Input: part model. Units: mm. Frame: model coordinates. Face numbers are marked on the shaded views. Give positions to 0.01 mm unless a question says otherwise; leave off trailing zeros. Write each loop counter-clockwise with the first axis right and the second up, starting at its lowest first coordinate (ties: lowest second). Pieces come first, ordered by that corner, then holes. Notation, with made-up numbers: (-37.75, -7.75) - (-11.75, -7.75) arc R15 cw to (-11.75, 15.25) - close; hole circle Ø4 at (-17, -19). An arc over 180 degrees is marked (long way). Use a Markdown table: item, result. Add a question column.
1. Section query A-A, the plane y = 0. Return loops of the section in (x, z), plus the area to 3 significant figures.
2. Pin query (flat end, axial travel): pin 1 (2 mm diameter, centred on x = -4.5, y = -12, fed in from -Z); pin 2 (1 mm diameter, centred on x = 3.5, z = -15, fed in from +Y); pin 3 (3 mm diameter, centred on x = 6.5, y = 30.5, fed in from -Z). Return the tip coordinate at first contact, or that it passes through.
3. Mould query, pull axis Y, two halves, no side actions, for the marked faces 1, 2 and 3. Classes: released by +Y, released by -Y, zero draft, split by the parting line, or undercut.
4. Section query C-C, the plane x = -4.5. Return loops of the section in (y, z), plus the area to 3 significant figures.
5. Material intervals for probe 1 along Y at (x, z) = (-1.5, 0); probe 2 along Y at (x, z) = (-6, -5); probe 3 along Z at (x, y) = (-6, -9.5), sorted ascending.
```python
from build123d import *

# Parameters (mm, degrees)
SKETCH1_R           = 39.5
SKETCH1_R_2         = 25
BOSS_EXTRUDE1_DEPTH = 8.75
FILLET1_R           = 3
CHAMFER1_SIZE       = 1.3


with BuildPart() as part:
    # Sketch1 → Boss-Extrude1 (new, symmetric)
    with BuildSketch(Plane(origin=(0, 0, 0), x_dir=(0, 0, -1), z_dir=(1, 0, 0))):
        Circle(SKETCH1_R)
        Circle(SKETCH1_R_2, mode=Mode.SUBTRACT)
    extrude(amount=BOSS_EXTRUDE1_DEPTH, both=True)

    # Fillet1
    fillet1_edges = [part.edges().sort_by_distance(p)[0] for p in [
        (-8.75, 0, 39.5),
        (8.75, 0, 39.5),
    ]]
    fillet(fillet1_edges, radius=FILLET1_R)

    # Chamfer1
    chamfer1_edges = [part.edges().sort_by_distance(p)[0] for p in [
        (-8.75, 0, 25),
        (8.75, 0, 25),
    ]]
    chamfer(chamfer1_edges, length=CHAMFER1_SIZE)


solid = part.part
```
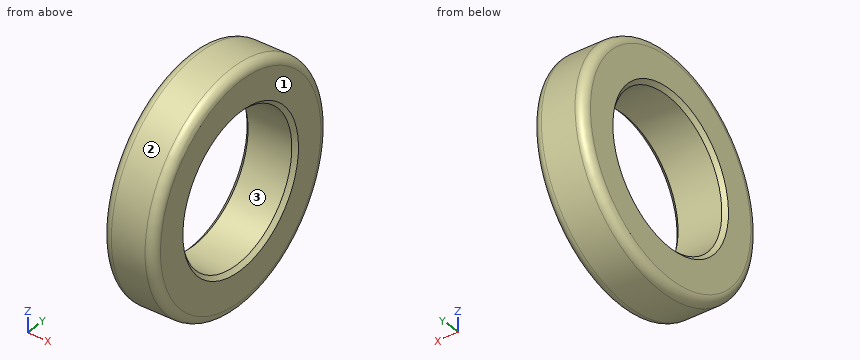
Result sheet:
| question | item | result |
|---|---|---|
| 1 | outline | (-8.75, -36.5) arc R3 ccw to (-5.75, -39.5) - (5.75, -39.5) arc R3 ccw to (8.75, -36.5) - (8.75, -26.3) - (7.45, -25) - (-7.45, -25) - (-8.75, -26.3) - close; (-8.75, 26.3) - (-7.45, 25) - (7.45, 25) - (8.75, 26.3) - (8.75, 36.5) arc R3 ccw to (5.75, 39.5) - (-5.75, 39.5) arc R3 ccw to (-8.75, 36.5) - close |
| 1 | area | 496 mm² |
| 2 | pin 1 | stops at z = -37.94 |
| 2 | pin 2 | stops at y = 36.74 |
| 2 | pin 3 | stops at z = -26.74 |
| 3 | face 1 | zero draft |
| 3 | face 2 | split by the parting line |
| 3 | face 3 | undercut |
| 4 | outline | circle Ø79 at (0, 0); hole circle Ø50 at (0, 0) |
| 4 | area | 2,940 mm² |
| 5 | probe 1 | y = -39.5 to -25, 25 to 39.5 |
| 5 | probe 2 | y = -39.17 to -24.49, 24.49 to 39.17 |
| 5 | probe 3 | z = -38.33 to -23.12, 23.12 to 38.33 |
